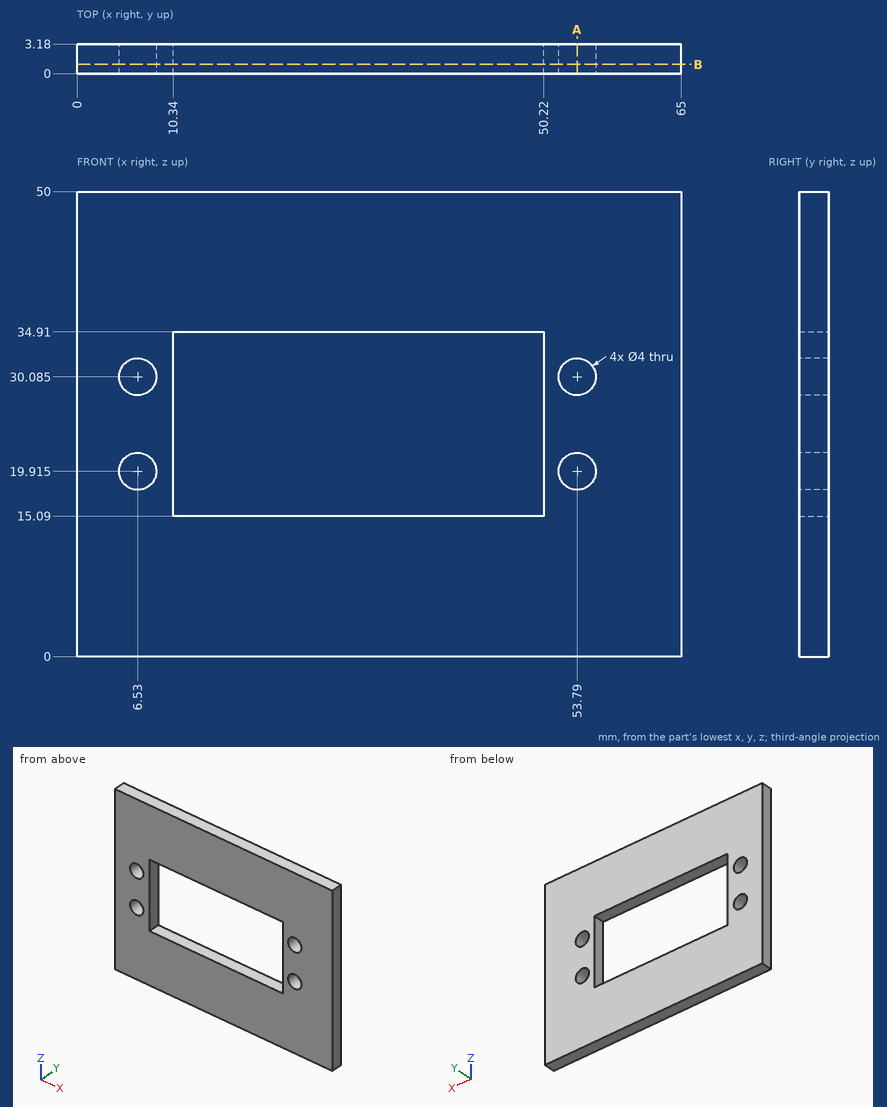
Geometry: see drawing. Coordinates: mm, zero at the bounding-box minimum. Coordinates: 2 decimals unless noted, no trailing zeros. Write each loop counter-clockwise with the first axis right and the second up, starting at its lowest first coordinate (ties: lowest second). Pieces come first, ordered by that corner, then holes. Notation, with made-up numbers: M -29.5,37 L 7.5,37 A16 cw 7.5,66 Z; hole C -11.5,89.25 d10. An arc over 180 degrees is marked long. Use CSV: the item, a comma, the result in double quotes. Start each with the question number.
1. Ray query, probe 1 along Z at (x, y) = (53.79, 2.2) (3 decimals); probe 2 along X at (y, z) = (0.2, 26); probe 3 along Z at (x, y) = (52, 0.25). Return the intervals inside material, ascending.
2. Cut plane A-A on x = 53.79. Return the cut outline in (y, z) (3 decimals).
3. First-contact query: P1, Ø3, axis at x = 53.79, z = 19.915, coming from the -Y side. Flat tip, straight axial feed; report the tip coordinate or a pass-through.
4. Cut plane B-B on y = 1. Return the cut outline in (x, z) (3 decimals).
Entries:
1,probe 1,"0 to 17.915, 21.915 to 28.085, 32.085 to 50"
1,probe 2,"0 to 10.34, 50.22 to 65"
1,probe 3,"0 to 19.02, 20.81 to 29.19, 30.98 to 50"
2,outline,"M 0,0 L 3.18,0 L 3.18,17.915 L 0,17.915 Z; M 0,21.915 L 3.18,21.915 L 3.18,28.085 L 0,28.085 Z; M 0,32.085 L 3.18,32.085 L 3.18,50 L 0,50 Z"
3,P1,"through"
4,outline,"M 0,0 L 65,0 L 65,50 L 0,50 Z; hole C 6.53,19.915 d4; hole C 6.53,30.085 d4; hole M 10.34,15.09 L 50.22,15.09 L 50.22,34.91 L 10.34,34.91 Z; hole C 53.79,19.915 d4; hole C 53.79,30.085 d4"
